Can you work these out from the model? Positions are in its coordinate system, mm. A direction names the side the tool comes from. Give positions to 0.01 mm unless a question says otherwise; leave off trailing zeros. Loops run counter-clockwise (first coordinate to the right, second up) from the corner with the lowest first, then second, coordinate; pieces in that order, holes last. Notation, with made-up numbers: (-33, 57.5) -> (-23, 57.5) arc R20 cw to (-23, 85.5) -> close; hole circle Ø7 at (-30.5, 42.25). An arc over 180 degrees is marked (long way). Return JSON: item names as keys, results as strings. Group by question number.
Q1. Which directions (+Z, -Z, +X, -X, +Y, -Y) give clear straight access to the entire face, cutting with the end or side of a thin tool? Please do faces 4 (the flat face through (39, -14, 15)), 5 (the flat face through (-1, 22.75, 10)), 6 (the flat face through (0, -21.25, -1)), 7 (the flat face through (1, 19, 0)), 8 (the flat face through (-16, -26, 12)).
Q2. I need wall thicknesses on line 1 along X through (y, z) = (5, 2.5); line 2 along X through (y, z) = (21.65, 8); line 3 along Y through (x, z) = (-29, 2). Which ranges of each line are inside material? Lowest first, please. Write a range as [from, to].
Q3. Will this pin go through, and if not, where does the flat tip stop? pin 1 (3 mm diameter, centred on x = -4, y = 15, fed in from -Z).
Q4. Thinking about a two-plate mould opening in X: for faces 1 (the cylindrical face through (24.01, 21.76, 10.08)), 2 (the flat face through (40, -2, 10)), 3 (the cylindrical face through (39.01, -9.25, 13.04)), which applies, pulls with the +X half, pulls with the -X half, needs draft (parallel to the pull), parting line crosses it, or undercut?
Q5. Suppose I cut it at A-A, the plane y = -15.5. Please give me the cut outline in (x, z), and give its area (3 significant figures).
Q6. Suppose I cut it at C-C, the plane z = 8. Please give me the cut outline in (x, y), and give its area (3 significant figures).
Q7. Suppose I cut it at B-B, the plane x = -21. Please give me the cut outline in (y, z), and give its area (3 significant figures).
Q8. Suppose I cut it at D-D, the plane y = -6.5. Please give me the cut outline in (x, z).
```python
from build123d import *

# Parameters (mm, degrees)
SKETCH_1_W           = 80
SKETCH_1_H           = 51.5
SKETCH_1_W_2         = 76
SKETCH_1_H_2         = 50.5
EXTRUDE_1_DEPTH      = 22
SKETCH_2_W           = 80
SKETCH_2_H           = 51.5
EXTRUDE_2_DEPTH      = 2
CUT_EXTRUDE_1_REACH  = 88.874
CUT_EXTRUDE_2_REACH  = 70.82
SKETCH_6_W           = 7.5
SKETCH_6_H           = 3.5
CUT_EXTRUDE_3_REACH  = 70.82
SKETCH_7_W           = 76
SKETCH_7_H           = 20
SKETCH_8_W           = 80
SKETCH_8_H           = 51.5
EXTRUDE_3_DEPTH      = 2
SKETCH_9_W           = 62
SKETCH_9_H           = 36
CUT_EXTRUDE_4_DEPTH  = 2
SKETCH_15_W          = 80
SKETCH_15_H          = 24
EXTRUDE_5_DEPTH      = 1
SKETCH_16_W          = 7.5
SKETCH_16_H          = 3.5
CUT_EXTRUDE_6_DEPTH  = 1
SKETCH_17_W          = 62
SKETCH_17_H          = 2
CUT_EXTRUDE_7_DEPTH  = 2
SKETCH_19_W          = 80
SKETCH_19_H          = 24
CUT_EXTRUDE_8_DEPTH  = 3
SKETCH_20_W          = 76
SKETCH_20_H          = 2
EXTRUDE_6_DEPTH      = 20
SKETCH_21_W          = 76
SKETCH_21_H          = 46
CUT_EXTRUDE_9_DEPTH  = 10
FILLET_1_R           = 1
SKETCH_22_R          = 4.5
CUT_EXTRUDE_10_DEPTH = 10
SKETCH_23_W          = 62
SKETCH_23_H          = 0.5
CUT_EXTRUDE_11_DEPTH = 10


with BuildPart() as part:
    # 草图1 → 凸台-拉伸1 (new body)
    with BuildSketch(Plane.XY):
        Rectangle(SKETCH_1_W, SKETCH_1_H)
        Rectangle(SKETCH_1_W_2, SKETCH_1_H_2, mode=Mode.SUBTRACT)
    extrude(amount=EXTRUDE_1_DEPTH)

    # 草图2 → 凸台-拉伸2 (add)
    with BuildSketch(Plane.XY.offset(22)):
        Rectangle(SKETCH_2_W, SKETCH_2_H)
    extrude(amount=-EXTRUDE_2_DEPTH)

    # 草图4 → 切除-拉伸1 (cut, up to next)
    with BuildSketch(Plane(origin=(40, 0, 0), x_dir=(0, 0, -1), z_dir=(1, 0, 0)), mode=Mode.PRIVATE) as cut_extrude_1_sk1:
        with BuildLine():
            Line((-11, -11.25), (-11, -17.25))
            ThreePointArc((-11, -17.25), (-13, -19.25), (-15, -17.25))
            Line((-15, -17.25), (-15, -11.25))
            ThreePointArc((-15, -11.25), (-13, -9.25), (-11, -11.25))
        make_face()
    cut_extrude_1_tool1 = extrude(cut_extrude_1_sk1.sketch, amount=-CUT_EXTRUDE_1_REACH, mode=Mode.PRIVATE) & part.part
    add(cut_extrude_1_tool1.solids().sort_by_distance((40, -14.25, 13))[0], mode=Mode.SUBTRACT)

    # 草图6 → 切除-拉伸2 (cut, up to next)
    with BuildSketch(Plane.XZ.offset(25.75), mode=Mode.PRIVATE) as cut_extrude_2_sk1:
        with Locations((-19.75, 12.25)):
            Rectangle(SKETCH_6_W, SKETCH_6_H)
    cut_extrude_2_tool1 = extrude(cut_extrude_2_sk1.sketch, amount=-CUT_EXTRUDE_2_REACH, mode=Mode.PRIVATE) & part.part
    add(cut_extrude_2_tool1.solids().sort_by_distance((-19.75, -25.75, 12.25))[0], mode=Mode.SUBTRACT)

    # 草图7 → 切除-拉伸3 (cut, up to next)
    with BuildSketch(Plane(origin=(0, 25.75, 0), x_dir=(1, 0, 0), z_dir=(0, 1, 0)), mode=Mode.PRIVATE) as cut_extrude_3_sk1:
        with Locations((0, -10)):
            Rectangle(SKETCH_7_W, SKETCH_7_H)
    cut_extrude_3_tool1 = extrude(cut_extrude_3_sk1.sketch, amount=-CUT_EXTRUDE_3_REACH, mode=Mode.PRIVATE) & part.part
    add(cut_extrude_3_tool1.solids().sort_by_distance((0, 25.75, 10))[0], mode=Mode.SUBTRACT)

    # 草图8 → 凸台-拉伸3 (add)
    with BuildSketch(Plane(origin=(0, 0, 0), x_dir=(-1, 0, 0), z_dir=(0, 0, -1))):
        Rectangle(SKETCH_8_W, SKETCH_8_H)
    extrude(amount=EXTRUDE_3_DEPTH)

    # 草图9 → 切除-拉伸4 (cut)
    with BuildSketch(Plane(origin=(0, 0, -2), x_dir=(-1, 0, 0), z_dir=(0, 0, -1))):
        with Locations((0, -1.25)):
            Rectangle(SKETCH_9_W, SKETCH_9_H)
    extrude(amount=-CUT_EXTRUDE_4_DEPTH, mode=Mode.SUBTRACT)

    # 草图15 → 凸台-拉伸5 (add)
    with BuildSketch(Plane.XZ.offset(25.75)):
        with Locations((0, 10)):
            Rectangle(SKETCH_15_W, SKETCH_15_H)
    extrude(amount=EXTRUDE_5_DEPTH)

    # 草图16 → 切除-拉伸6 (cut)
    with BuildSketch(Plane(origin=(0, -25.75, 0), x_dir=(1, 0, 0), z_dir=(0, 1, 0))):
        with Locations((-19.75, -12.25)):
            Rectangle(SKETCH_16_W, SKETCH_16_H)
    extrude(amount=-CUT_EXTRUDE_6_DEPTH, mode=Mode.SUBTRACT)

    # 草图17 → 切除-拉伸7 (cut)
    with BuildSketch(Plane(origin=(0, 0, -2), x_dir=(-1, 0, 0), z_dir=(0, 0, -1))):
        with Locations((0, -20.25)):
            Rectangle(SKETCH_17_W, SKETCH_17_H)
    extrude(amount=-CUT_EXTRUDE_7_DEPTH, mode=Mode.SUBTRACT)

    # 草图19 → 切除-拉伸8 (cut)
    with BuildSketch(Plane(origin=(0, 25.75, 0), x_dir=(1, 0, 0), z_dir=(0, 1, 0))):
        with Locations((0, -10)):
            Rectangle(SKETCH_19_W, SKETCH_19_H)
    extrude(amount=-CUT_EXTRUDE_8_DEPTH, mode=Mode.SUBTRACT)

    # 草图20 → 凸台-拉伸6 (add)
    with BuildSketch(Plane(origin=(0, 0, 20), x_dir=(-1, 0, 0), z_dir=(0, 0, -1))):
        with Locations((0, 21.75)):
            Rectangle(SKETCH_20_W, SKETCH_20_H)
    extrude(amount=EXTRUDE_6_DEPTH)

    # 草图21 → 切除-拉伸9 (cut)
    with BuildSketch(Plane(origin=(0, 0, 20), x_dir=(-1, 0, 0), z_dir=(0, 0, -1))):
        with Locations((0, -2.25)):
            Rectangle(SKETCH_21_W, SKETCH_21_H)
    extrude(amount=-CUT_EXTRUDE_9_DEPTH, mode=Mode.SUBTRACT)

    # 圆角1
    fillet_1_edges = [part.edges().sort_by_distance(p)[0] for p in [
        (-40, -26.75, 10),
        (0, -26.75, -2),
        (40, -26.75, 10),
        (40, -2, -2),
        (-40, 22.75, 10),
        (0, 22.75, -2),
        (40, 22.75, 10),
        (-40, -2, -2),
    ]]
    fillet(fillet_1_edges, radius=FILLET_1_R)

    # 草图22 → 切除-拉伸10 (cut)
    with BuildSketch(Plane(origin=(0, 22.75, 0), x_dir=(1, 0, 0), z_dir=(0, 1, 0))):
        with Locations(Location((28, -8, 0), (0, 0, 270))):
            Circle(SKETCH_22_R)
    extrude(amount=-CUT_EXTRUDE_10_DEPTH, mode=Mode.SUBTRACT)

    # 草图23 → 切除-拉伸11 (cut)
    with BuildSketch(Plane(origin=(0, 0, -2), x_dir=(-1, 0, 0), z_dir=(0, 0, -1))):
        with Locations((0, 17)):
            Rectangle(SKETCH_23_W, SKETCH_23_H)
    extrude(amount=-CUT_EXTRUDE_11_DEPTH, mode=Mode.SUBTRACT)


solid = part.part
```
Ans:
{
 "1": {"face 4": "+X", "face 5": "+Z, -Z, +X, -X, +Y", "face 6": "+Z, -Z", "face 7": "+Z", "face 8": "-Y"},
 "2": {"line 1": "x = [-40, -38], [38, 40]", "line 2": "x = [-40, 23.5], [32.5, 40]", "line 3": "y = [-26.75, -25.25], [20.75, 22.75]"},
 "3": {"pin 1": "passes through"},
 "4": {"face 1": "undercut", "face 2": "pulls with the +X half", "face 3": "needs draft"},
 "5": {"outline": "(-40, -1) arc R1 ccw to (-39, -2) -> (-31, -2) -> (-31, 0) -> (-38, 0) -> (-38, 22) -> (-40, 22) -> close; (31, -2) -> (39, -2) arc R1 ccw to (40, -1) -> (40, 11) -> (38, 11) -> (38, 0) -> (31, 0) -> close; (38, 15) -> (40, 15) -> (40, 22) -> (38, 22) -> close", "area": "116 mm^2"},
 "6": {"outline": "(-40, -25.75) arc R1 ccw to (-39, -26.75) -> (39, -26.75) arc R1 ccw to (40, -25.75) -> (40, 21.75) arc R1 ccw to (39, 22.75) -> (32.5, 22.75) -> (32.5, 20.75) -> (38, 20.75) -> (38, -25.25) -> (-38, -25.25) -> (-38, 20.75) -> (23.5, 20.75) -> (23.5, 22.75) -> (-39, 22.75) arc R1 ccw to (-40, 21.75) -> close", "area": "445 mm^2"},
 "7": {"outline": "(-26.75, -1) arc R1 ccw to (-25.75, -2) -> (-21.25, -2) -> (-21.25, 0) -> (-25.25, 0) -> (-25.25, 10.5) -> (-26.75, 10.5) -> close; (-26.75, 14) -> (-25.25, 14) -> (-25.25, 22) -> (-26.75, 22) -> close; (17.25, -2) -> (21.75, -2) arc R1 ccw to (22.75, -1) -> (22.75, 22) -> (20.75, 22) -> (20.75, 0) -> (17.25, 0) -> close", "area": "93.3 mm^2"},
 "8": {"outline": "(-40, -1) arc R1 ccw to (-39, -2) -> (-31, -2) -> (-31, 0) -> (-38, 0) -> (-38, 22) -> (-40, 22) -> close; (31, -2) -> (39, -2) arc R1 ccw to (40, -1) -> (40, 22) -> (38, 22) -> (38, 0) -> (31, 0) -> close"}
}
